from build123d import *

# Parameters (mm, degrees)
F1_DEPTH = 6.35
F2_R     = 7.62


with BuildPart() as f1:
    # F0 (on Front) → F1 (new body)
    with BuildSketch(Plane.XZ):
        with BuildLine():
            Line((-6.35, 0), (0, 0))
            Line((0, 0), (0, 7.62))
            Line((0, 7.62), (16.51, 7.62))
            Line((16.51, 7.62), (16.51, 0))
            Line((16.51, 0), (22.86, 0))
            Line((22.86, 0), (35.56, 20.32))
            ThreePointArc((35.56, 20.32), (48.26, 33.02), (35.56, 45.72))
            Line((35.56, 45.72), (-19.05, 45.72))
            ThreePointArc((-19.05, 45.72), (-31.75, 33.02), (-19.05, 20.32))
            Line((-19.05, 20.32), (-6.35, 0))
        make_face()
        with BuildLine():
            Line((35.56, 26.67), (-19.05, 26.67))
            ThreePointArc((-19.05, 26.67), (-25.4, 33.02), (-19.05, 39.37))
            Line((-19.05, 39.37), (35.56, 39.37))
            ThreePointArc((35.56, 39.37), (41.91, 33.02), (35.56, 26.67))
        make_face(mode=Mode.SUBTRACT)
    extrude(amount=F1_DEPTH)

    # F2
    f2_edges = [f1.edges().sort_by_distance(p)[0] for p in [
        (22.86, -3.175, 0),
        (-6.35, -3.175, 0),
        (35.56, -3.175, 20.32),
        (-19.05, -3.175, 20.32),
    ]]
    fillet(f2_edges, radius=F2_R)


solid = f1.part
The listing builds one solid part. Answer for the finished solid, in the listing's coordinates (mm). A direction names the side the tool comes from. Give positions to 0.01 mm unless a question says otherwise; leave off trailing zeros. Write each loop counter-clockwise with the first axis right and the second up, starting at its lowest first coordinate (ties: lowest second). Pieces come first, ordered by that corner, then holes.
Item 1: Which of the six approach directions +Z, -Z, +X, -X, +Y, -Y give full straight-line access (tool end or side, diameter ignored) to faces 1 (the flat face through (16.51, -3, 4)), 2 (the flat face through (9, -3, 26.67)), 3 (the flat face through (18, -3, 0))?
Item 2: Flat-ended cylindrical pins translate along their axes: P1, Ø1, axis at x = 32.5, y = -3.5, coming from the -Z side; P2, Ø3, axis at y = -2.5, z = 5, coming from the +X side; P3, Ø3, axis at y = -3, z = 2.5, coming from the -X side. Find the tip coordinate at first contact, or state that the pin passes through.
Item 3: Section A-A, the plane x = -11.5 is taken. Write down the section's boundary in (y, z), plus the area to 3 significant figures.
Item 4: Section B-B, the plane z = 29 is taken. Write down the section's boundary in (x, y), plus the area to 3 significant figures.
Item 5: Determine the mould class of faces 4 (the flat face through (8, -6.35, 23)), 5 (the cylindrical face through (22.283, -3.219, 0.929)), 6 (the cylindrical face through (41.91, -3.13, 33.16)) for opening direction Z: released by +Z, released by -Z, zero draft, split by the parting line, or undercut.
Item 6: Find the intervals of material crossed by line 1 along Z through (x, y) = (7, -0.25); line 2 along X through (y, z) = (-0.25, 33); line 3 along X through (y, z) = (-1.5, 7.5), in increasing order.
Item 7: Section D-D, the plane z = 10 is taken. Write down the section's boundary in (x, y).
Item 8: Section C-C, the plane y = -4.25 is taken. Write down the section's boundary in (x, z), plus the area to 3 significant figures.
Completed:
1. face 1: -Z, +Y, -Y
1. face 2: +Y, -Y
1. face 3: -Z, +X, -X, +Y, -Y
2. P1: stops at z = 14.62
2. P2: stops at x = 26.92
2. P3: stops at x = -8.85
3. outline: (-6.35, 8.24) - (0, 8.24) - (0, 26.67) - (-6.35, 26.67) - close; (-6.35, 39.37) - (0, 39.37) - (0, 45.72) - (-6.35, 45.72) - close
3. area: 157 mm2
4. outline: (-31.1, -6.35) - (-23.97, -6.35) - (-23.97, 0) - (-31.1, 0) - close; (40.48, -6.35) - (47.61, -6.35) - (47.61, 0) - (40.48, 0) - close
4. area: 90.6 mm2
5. face 4: zero draft
5. face 5: released by -Z
5. face 6: undercut
6. line 1: z = 7.62 to 26.67, 39.37 to 45.72
6. line 2: x = -31.75 to -25.4, 41.91 to 48.26
6. line 3: x = -11.04 to 0, 16.51 to 27.55
7. outline: (-12.6, -6.35) - (29.11, -6.35) - (29.11, 0) - (-12.6, 0) - close
8. outline: (-21.89, 20.64) arc R7.62 cw to (-17.13, 17.25) - (-8.59, 3.58) arc R7.62 ccw to (-2.13, 0) - (0, 0) - (0, 7.62) - (16.51, 7.62) - (16.51, 0) - (18.64, 0) arc R7.62 ccw to (25.1, 3.58) - (33.64, 17.25) arc R7.62 cw to (38.4, 20.64) arc R12.7 ccw to (35.56, 45.72) - (-19.05, 45.72) arc R12.7 ccw to start; hole (-19.05, 26.67) - (35.56, 26.67) arc R6.35 ccw to (35.56, 39.37) - (-19.05, 39.37) arc R6.35 ccw to start
8. area: 1,800 mm2
